```python
from build123d import *

# Parameters (mm, degrees)
SKETCH_1_R          = 20
SKETCH_1_W          = 45
SKETCH_1_H          = 40
EXTRUDE_1_DEPTH     = 3
SKETCH_3_R          = 1.275
CUT_EXTRUDE_3_DEPTH = 4
SKETCH_6_R          = 7.025
CUT_EXTRUDE_6_DEPTH = 4
FILLET_1_R          = 2
SKETCH_7_R          = 1.525
CUT_EXTRUDE_7_DEPTH = 4
CUT_EXTRUDE_8_DEPTH = 10


with BuildPart() as part:
    # 草图1 → 凸台-拉伸1 (new body)
    with BuildSketch(Plane(origin=(0, 0, 0), x_dir=(1, 0, 0), z_dir=(0, 1, 0))):
        with Locations((-22.5, 0)):
            Circle(SKETCH_1_R)
        Rectangle(SKETCH_1_W, SKETCH_1_H)
    extrude(amount=EXTRUDE_1_DEPTH)

    # 草图3 → 切除-拉伸3 (cut, through all)
    with BuildSketch(Plane(origin=(0, 0, 0), x_dir=(1, 0, 0), z_dir=(0, 1, 0))):
        with Locations((-36, 0)):
            Circle(SKETCH_3_R)
        with Locations((-29.25, 11.691342951)):
            Circle(SKETCH_3_R)
        with Locations((-15.75, 11.691342951)):
            Circle(SKETCH_3_R)
        with Locations((-9, 0)):
            Circle(SKETCH_3_R)
        with Locations((-15.75, -11.691342951)):
            Circle(SKETCH_3_R)
        with Locations((-29.25, -11.691342951)):
            Circle(SKETCH_3_R)
    extrude(amount=CUT_EXTRUDE_3_DEPTH, mode=Mode.SUBTRACT)

    # 草图6 → 切除-拉伸6 (cut, through all)
    with BuildSketch(Plane(origin=(0, 3, 0), x_dir=(1, 0, 0), z_dir=(0, 1, 0))):
        with Locations((-22.5, 0)):
            Circle(SKETCH_6_R)
    extrude(amount=-CUT_EXTRUDE_6_DEPTH, mode=Mode.SUBTRACT)

    # 圆角1
    fillet_1_edges = [part.edges().sort_by_distance(p)[0] for p in [
        (22.5, 1.5, -20),
        (22.5, 1.5, 20),
    ]]
    fillet(fillet_1_edges, radius=FILLET_1_R)

    # 草图7 → 切除-拉伸7 (cut, through all)
    with BuildSketch(Plane(origin=(0, 3, 0), x_dir=(1, 0, 0), z_dir=(0, 1, 0))):
        with Locations((19, -14)):
            Circle(SKETCH_7_R)
        with Locations((19, 14)):
            Circle(SKETCH_7_R)
    extrude(amount=-CUT_EXTRUDE_7_DEPTH, mode=Mode.SUBTRACT)

    # 草图8 → 切除-拉伸8 (cut)
    with BuildSketch(Plane(origin=(0, 3, 0), x_dir=(1, 0, 0), z_dir=(0, 1, 0))):
        with BuildLine():
            Line((-0.51493536, -4.000000002), (11.500000002, -4.000000002))
            ThreePointArc((11.500000002, -4.000000002), (12.207106783, -4.29289322), (12.500000002, -5.000000002))
            Line((12.500000002, -5.000000002), (12.500000002, -11.000000002))
            ThreePointArc((12.500000002, -11.000000002), (12.207106783, -11.707106783), (11.500000002, -12.000000002))
            Line((11.500000002, -12.000000002), (1.461970397, -12.000000002))
            ThreePointArc((1.461970397, -12.000000002), (0.782245955, -11.733467577), (0.464858721, -11.075949369))
            ThreePointArc((0.464858721, -11.075949369), (-0.111079243, -8.192615452), (-1.361902294, -5.531645571))
            ThreePointArc((-1.361902294, -5.531645571), (-1.390048372, -4.516081398), (-0.51493536, -4.000000002))
        make_face()
    cut_extrude_8 = extrude(amount=-CUT_EXTRUDE_8_DEPTH, mode=Mode.SUBTRACT)

    # 镜向1: 切除-拉伸8 across plane
    add(cut_extrude_8.mirror(Plane.XY), mode=Mode.SUBTRACT)


solid = part.part
```
Verification items for the finished model (mm, model axes). A direction names the side the tool comes from. Give positions to 0.01 mm unless a question says otherwise; leave off trailing zeros. Order: outer loops, then holes, each group sorted by start corner. A loop starts at its lowest first (then second) coordinate and runs counter-clockwise, first axis right, second up. Notation, with made-up numbers: M -36.75,33.25 L -14.75,33.25 A3 ccw -14.75,37.25 Z; hole C 7,-1 d5. An arc over 180 degrees is marked long. Return JSON: item names as keys, results as strings. Group by question number.
1) Section check A-A on x = 19. Record the cut outline in (y, z) (3 decimals).
2) Section check C-C on x = -19.5. Record the cut outline in (y, z).
3) Section check B-B on z = 0. Record the cut outline in (x, y) (3 decimals), and give its area (3 significant figures).
4) Access from +Z, -Z, +X, -X, +Y, -Y to the whole of each face (thin tool, end or side, straight path). Record for faces 4 (the face through (-1, 1, 20)), 5 (the face through (7, 2, 12)).
5) Mould release check, pull along X, two halves, no side actions. Record for faces 1 (the face through (-0.1, 1.52, 8.23)), 2 (the face through (-10.5, 0, -0.3)), 3 (the face through (22.5, 1, 0)): pulls with the +X half, pulls with the -X half, needs draft (parallel to the pull), parting line crosses it, or undercut.
6) Scan lines: line 1 (Z direction, x = 5.5, y = 2.6); line 2 (Z direction, x = -9, y = 2.15) (3 decimals); line 3 (Z direction, x = 19, y = 2.05) (3 decimals). Record each from-to range of solid material in increasing order.
7) Section check D-D on z = 14. Record the cut outline in (x, y) (3 decimals).
8) Go/stop test with flat-tipped pins: pin 1 Ø0.9 at (y, z) = (1, 7) entering from -X; pin 2 Ø0.9 at (y, z) = (2, -7.5) entering from -X. Record where each tip stops, or that it passes through.
Answer block:
{
 "1": {"outline": "M 0,-20 L 3,-20 L 3,-15.525 L 0,-15.525 Z; M 0,-12.475 L 3,-12.475 L 3,12.475 L 0,12.475 Z; M 0,15.525 L 3,15.525 L 3,20 L 0,20 Z"},
 "2": {"outline": "M 0,-20 L 3,-20 L 3,-6.35 L 0,-6.35 Z; M 0,6.35 L 3,6.35 L 3,20 L 0,20 Z"},
 "3": {"outline": "M -42.5,0 L -37.275,0 L -37.275,3 L -42.5,3 Z; M -34.725,0 L -29.525,0 L -29.525,3 L -34.725,3 Z; M -15.475,0 L -10.275,0 L -10.275,3 L -15.475,3 Z; M -7.725,0 L 22.5,0 L 22.5,3 L -7.725,3 Z", "area": "138 mm^2"},
 "4": {"face 4": "+Z, +X, -X, +Y, -Y", "face 5": "+Y, -Y"},
 "5": {"face 1": "undercut", "face 2": "needs draft", "face 3": "pulls with the +X half"},
 "6": {"line 1": "z = -20 to -12, -4 to 4, 12 to 20", "line 2": "z = -20 to -1.275, 1.275 to 20", "line 3": "z = -20 to -15.525, -12.475 to 12.475, 15.525 to 20"},
 "7": {"outline": "M -36.783,0 L 17.475,0 L 17.475,3 L -36.783,3 Z; M 20.525,0 L 22.5,0 L 22.5,3 L 20.525,3 Z"},
 "8": {"pin 1": "stops at x = -41.4", "pin 2": "stops at x = -41.22"}
}
